The listing builds one solid part. Answer for the finished solid, in the listing's coordinates (mm). Face numbers are marked on the shaded views. Coordinates: 2 decimals unless noted, no trailing zeros. Loops run counter-clockwise (first coordinate to the right, second up) from the corner with the lowest first, then second, coordinate; pieces in that order, holes last. Notation, with made-up numbers: (15, 56) - (61, 56) arc R17 cw to (61, 63) - close; hole circle Ø7 at (-27, 86). An arc over 180 degrees is marked (long way). Write each question's results on one line, items separated by ' | '. Start each with the question number.
(1) Find section C-C on x = 20. Determine the outline of the cut face in (y, z).
(2) Find section D-D on z = -36. Determine the outline of the cut face in (x, y).
(3) Find section A-A on x = 36. Determine the outline of the cut face in (y, z), then the cut area to 3 significant figures.
(4) Consider line 1 (X direction, y = 4.25, z = -4); line 2 (Z direction, x = 37, y = 7.75); line 3 (X direction, y = 3.15, z = -20). Determine where each line is inside the solid, lowest interval first. Write a range as from..to.
(5) Given pin 1 Ø4 at (x, z) = (20, -20) entering from +Y, flat-ended and moving along its own axis, determine where the tip first touches the part or whether it passes through.
(6) Find section B-B on y = 5.25. Determine the outline of the cut face in (x, z) (1 decimal), then the cut area to 3 significant figures.
(7) Determine the mould class of the marked faces 1, 2, 3 and 4 for opening direction X: released by +X, released by -X, zero draft, split by the parting line, or undercut.
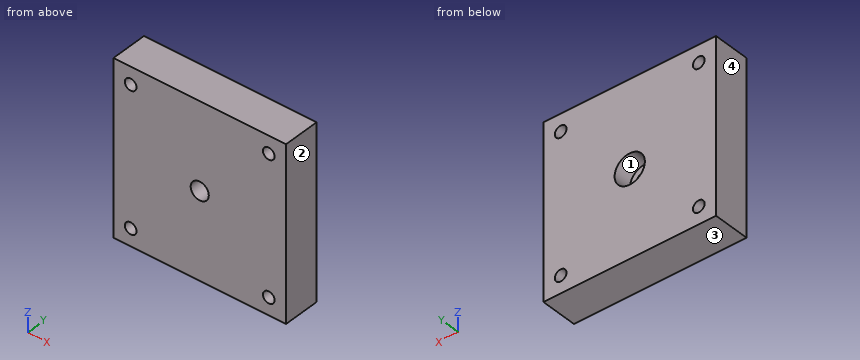
from build123d import *

# Parameters (mm, degrees)
SKETCH1_W           = 40
SKETCH1_H           = 40
BOSS_EXTRUDE1_DEPTH = 8.5
SKETCH2_R           = 1.3525
SKETCH2_R_2         = 2.1
CUT_EXTRUDE1_DEPTH  = 9.5
SKETCH3_R           = 3.5
CUT_EXTRUDE2_DEPTH  = 4.25


with BuildPart() as part:
    # Sketch1 → Boss-Extrude1 (new body)
    with BuildSketch(Plane(origin=(0, 0, 0), x_dir=(1, 0, 0), z_dir=(0, 1, 0))):
        with Locations((20, 20)):
            Rectangle(SKETCH1_W, SKETCH1_H)
    extrude(amount=BOSS_EXTRUDE1_DEPTH)

    # Sketch2 → Cut-Extrude1 (cut, through all)
    with BuildSketch(Plane(origin=(0, 8.5, 0), x_dir=(1, 0, 0), z_dir=(0, 1, 0))):
        with Locations((4, 4)):
            Circle(SKETCH2_R)
        with Locations((36, 4)):
            Circle(SKETCH2_R)
        with Locations((36, 36)):
            Circle(SKETCH2_R)
        with Locations((4, 36)):
            Circle(SKETCH2_R)
        with Locations((20, 20)):
            Circle(SKETCH2_R_2)
    extrude(amount=-CUT_EXTRUDE1_DEPTH, mode=Mode.SUBTRACT)

    # Sketch3 → Cut-Extrude2 (cut)
    with BuildSketch(Plane(origin=(0, 8.5, 0), x_dir=(1, 0, 0), z_dir=(0, 1, 0))):
        with Locations((20, 20)):
            Circle(SKETCH3_R)
    extrude(amount=-CUT_EXTRUDE2_DEPTH, mode=Mode.SUBTRACT)


solid = part.part
Values:
1) outline: (0, -40) - (8.5, -40) - (8.5, -23.5) - (4.25, -23.5) - (4.25, -22.1) - (0, -22.1) - close; (0, -17.9) - (4.25, -17.9) - (4.25, -16.5) - (8.5, -16.5) - (8.5, 0) - (0, 0) - close
2) outline: (0, 0) - (2.65, 0) - (2.65, 8.5) - (0, 8.5) - close; (5.35, 0) - (34.65, 0) - (34.65, 8.5) - (5.35, 8.5) - close; (37.35, 0) - (40, 0) - (40, 8.5) - (37.35, 8.5) - close
3) outline: (0, -40) - (8.5, -40) - (8.5, -37.35) - (0, -37.35) - close; (0, -34.65) - (8.5, -34.65) - (8.5, -5.35) - (0, -5.35) - close; (0, -2.65) - (8.5, -2.65) - (8.5, 0) - (0, 0) - close | area: 294 mm²
4) line 1: x = 0..2.65, 5.35..34.65, 37.35..40 | line 2: z = -40..-36.91, -35.09..-4.91, -3.09..0 | line 3: x = 0..17.9, 22.1..40
5) pin 1: passes through
6) outline: (0, -40) - (40, -40) - (40, 0) - (0, 0) - close; hole circle Ø2.7 at (4, -36); hole circle Ø2.7 at (4, -4); hole circle Ø7 at (20, -20); hole circle Ø2.7 at (36, -36); hole circle Ø2.7 at (36, -4) | area: 1,540 mm²
7) face 1: undercut | face 2: released by +X | face 3: zero draft | face 4: released by -X
